from build123d import *

# Parameters (mm, degrees)
BOSS_EXTRUDE1_DEPTH      = 457.2
BOSS_EXTRUDE1_DEPTH_BACK = 457.2
SKETCH5_R                = 3.81
CUT_EXTRUDE1_DEPTH       = 459.081095441
CUT_EXTRUDE2_DEPTH       = 459.081095441
CUT_EXTRUDE4_DEPTH       = 618.719010665
CUT_EXTRUDE4_DEPTH_BACK  = 618.719010665


with BuildPart() as part:
    # Sketch4 → Boss-Extrude1 (new, two sides: drawn at the far end of the back side and taken through both)
    with BuildSketch(Plane(origin=(0, 0, 0), x_dir=(0, 0, -1), z_dir=(1, 0, 0)).offset(-BOSS_EXTRUDE1_DEPTH_BACK)):
        with BuildLine():
            Line((12.7, -11.43), (12.7, 11.43))
            ThreePointArc((12.7, 11.43), (12.328025612, 12.328025612), (11.43, 12.7))
            Line((11.43, 12.7), (-11.43, 12.7))
            ThreePointArc((-11.43, 12.7), (-12.328025612, 12.328025612), (-12.7, 11.43))
            Line((-12.7, 11.43), (-12.7, -11.43))
            ThreePointArc((-12.7, -11.43), (-12.328025612, -12.328025612), (-11.43, -12.7))
            Line((-11.43, -12.7), (11.43, -12.7))
            ThreePointArc((11.43, -12.7), (12.328025612, -12.328025612), (12.7, -11.43))
        make_face()
        with BuildLine():
            Line((10.5918, 9.53262), (10.5918, -9.53262))
            ThreePointArc((10.5918, -9.53262), (10.28157336, -10.28157336), (9.53262, -10.5918))
            Line((9.53262, -10.5918), (-9.53262, -10.5918))
            ThreePointArc((-9.53262, -10.5918), (-10.28157336, -10.28157336), (-10.5918, -9.53262))
            Line((-10.5918, -9.53262), (-10.5918, 9.53262))
            ThreePointArc((-10.5918, 9.53262), (-10.28157336, 10.28157336), (-9.53262, 10.5918))
            Line((-9.53262, 10.5918), (9.53262, 10.5918))
            ThreePointArc((9.53262, 10.5918), (10.28157336, 10.28157336), (10.5918, 9.53262))
        make_face(mode=Mode.SUBTRACT)
    extrude(amount=BOSS_EXTRUDE1_DEPTH + BOSS_EXTRUDE1_DEPTH_BACK)

    # Sketch5 → Cut-Extrude1 (cut, through all)
    with BuildSketch(Plane(origin=(0, 12.7, 0), x_dir=(1, 0, 0), z_dir=(0, 1, 0))):
        with Locations(Location((-444.5, 0, 0), (0, 0, 270))):
            Circle(SKETCH5_R)
    extrude(amount=-CUT_EXTRUDE1_DEPTH, mode=Mode.SUBTRACT)

    # Sketch7 → Cut-Extrude2 (cut, through all)
    with BuildSketch(Plane(origin=(0, 12.7, 0), x_dir=(1, 0, 0), z_dir=(0, 1, 0))):
        Polygon((457.2, 12.7), (442.535303163, -12.7), (457.2, -12.7), align=None)
    extrude(amount=-CUT_EXTRUDE2_DEPTH, mode=Mode.SUBTRACT)

    # Sketch8 → Cut-Extrude4 (cut, two sides: drawn at the far end of the back side and taken through both)
    with BuildSketch(Plane(origin=(119.799261314, 0, -207.498407305), x_dir=(0, 1, 0), z_dir=(0.5000000000000046, 0, -0.866025403784436)).offset(-CUT_EXTRUDE4_DEPTH_BACK)):
        with BuildLine():
            Line((1441.154483305, 1098.308705448), (12.7, 389.59681461))
            ThreePointArc((12.7, 389.59681461), (0, 386.619482961), (-12.7, 389.59681461))
            Line((-12.7, 389.59681461), (-1441.154483305, 1098.308705448))
            Line((-1441.154483305, 1098.308705448), (-1441.154483305, 4287.512214218))
            Line((-1441.154483305, 4287.512214218), (1441.154483305, 4287.512214218))
            Line((1441.154483305, 4287.512214218), (1441.154483305, 1098.308705448))
        make_face()
    extrude(amount=CUT_EXTRUDE4_DEPTH + CUT_EXTRUDE4_DEPTH_BACK, mode=Mode.SUBTRACT)


solid = part.part
The model under review builds one solid part; all positions refer to its coordinate system, in mm. A direction names the side the tool comes from. Round coordinates to 2 decimals unless told otherwise and drop trailing zeros. Order: outer loops, then holes, each group sorted by start corner. A loop starts at its lowest first (then second) coordinate and runs counter-clockwise, first axis right, second up. Notation, with made-up numbers: (-2.75, -24.5) -> (29.25, -24.5) arc R23 cw to (29.25, 14.5) -> close; hole circle Ø2 at (66.5, -29). An arc over 180 degrees is marked (long way). Return JSON: item names as keys, results as strings.
1. Take a section at B-B (y = 3.75). Write out the cut boundary in (x, z), then the cut area to 3 significant figures.
Answer block:
{"outline": "(-457.2, -12.7) -> (454.05, -12.7) -> (452.83, -10.59) -> (-457.2, -10.59) -> close; (-457.2, 10.59) -> (440.6, 10.59) -> (439.38, 12.7) -> (-457.2, 12.7) -> close", "area": "3,810 mm²"}
2. For faces 5 (the face through (-7, -12.7, 0)), 6 (the face through (-8, 0, -10.592)), list the 3-axis set-ups (+Z, -Z, +X, -X, +Y, -Y) from which the entire face can be reached by the end or side of a thin tool; tool diameter is ignored.
Answer block:
{"face 5": "+Z, -Z, +X, -X, -Y", "face 6": "+X, -X"}
3. Take a section at A-A (x = 352.5). Write out the cut boundary in (y, z), then the cut area to 3 significant figures.
Answer block:
{"outline": "(-12.7, -11.43) arc R1.27 ccw to (-11.43, -12.7) -> (11.43, -12.7) arc R1.27 ccw to (12.7, -11.43) -> (12.7, 11.43) arc R1.27 ccw to (11.43, 12.7) -> (-11.43, 12.7) arc R1.27 ccw to (-12.7, 11.43) -> close; hole (-10.59, -9.53) arc R1.06 ccw to (-9.53, -10.59) -> (9.53, -10.59) arc R1.06 ccw to (10.59, -9.53) -> (10.59, 9.53) arc R1.06 ccw to (9.53, 10.59) -> (-9.53, 10.59) arc R1.06 ccw to (-10.59, 9.53) -> close", "area": "196 mm²"}
4. Insertion check: P1, Ø10, axis at x = -444.5, z = 0, coming from the -Y side. The pin has a flat end and moves straight along its axis. Give the tip position at first contact, or say it passes through.
Answer block:
{"P1": "stops at y = -12.7"}
5. For L1, parallel to Z at x = -368, y = 9.75; L2, parallel to Y at x = 251.5, z = -7; L3, parallel to Z at x = -444.5, y = -11.7, list the stretches that pass through material, from the lowest coordinate up. Write a range as [from, to].
Answer block:
{"L1": "z = [-12.7, -10.57], [10.57, 12.7]", "L2": "y = [-12.7, -10.59], [10.59, 12.7]", "L3": "z = [-12.67, -3.81], [3.81, 12.67]"}
6. The part is to be moulded in two halves that separate along Y. For faces 1 (the face through (-14, 0, 10.592)), 2 (the face through (-7, 12.7, 0)), 3 (the face through (-7, 0, -12.7)), 4 (the face through (-8, 10.592, 0)), say which applies: +Y half, -Y half, draft (parallel to the pull), parting line (faces both ways), or undercut.
Answer block:
{"face 1": "undercut", "face 2": "+Y half", "face 3": "draft", "face 4": "undercut"}
